The drawing under review shows one solid part. Ordinate dimensions are in mm from its lowest x, y, z. A direction names the side the tool comes from. Coordinates: 2 decimals unless noted, no trailing zeros. Loops run counter-clockwise (first coordinate to the right, second up) from the corner with the lowest first, then second, coordinate; pieces in that order, holes last. Notation, with made-up numbers: M -27,34.5 L 11,34.5 A34 cw 11,69.5 Z; hole C -7,11.25 d3. An arc over 180 degrees is marked long. Return JSON: item names as keys, results as strings.
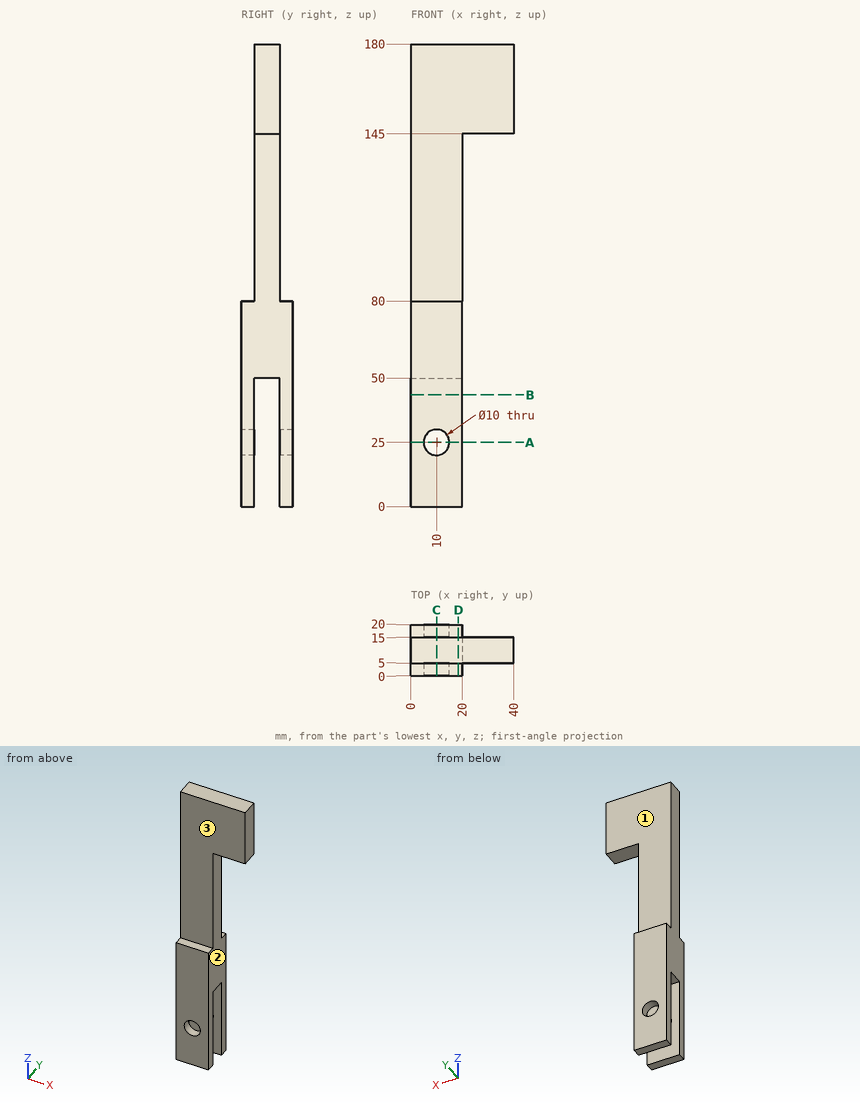
1. Add section A-A on z = 25. Give the boundary of the cut face in (x, y).
Check values:
{"outline": "M 0,0 L 5,0 L 5,5 L 0,5 Z; M 0,15 L 5,15 L 5,20 L 0,20 Z; M 15,0 L 20,0 L 20,5 L 15,5 Z; M 15,15 L 20,15 L 20,20 L 15,20 Z"}
2. Insertion check: pin 1 Ø2.5 at (x, y) = (10, 2.5) entering from +Z; pin 2 Ø11 at (x, y) = (30.5, 8) entering from -Z; pin 3 Ø3 at (y, z) = (5, 99) entering from +X. Each pin has a flat end and moves straight along its axis. Give the tip position at first contact, or say it passes through.
Check values:
{"pin 1": "z = 80", "pin 2": "z = 145", "pin 3": "x = 20"}
3. Add section C-C on x = 10. Give the boundary of the cut face in (y, z).
Check values:
{"outline": "M 0,0 L 5,0 L 5,20 L 0,20 Z; M 0,30 L 5,30 L 5,50 L 15,50 L 15,30 L 20,30 L 20,80 L 15,80 L 15,180 L 5,180 L 5,80 L 0,80 Z; M 15,0 L 20,0 L 20,20 L 15,20 Z"}
4. Machinability: for the marked faces 1, 2 and 3, which of the approach directions +Z, -Z, +X, -X, +Y, -Y give a long, thin tool a straight path to every point of the face, cutting with its end or side? Answer none if there is none.
Check values:
{"face 1": "+Z, +X, -X, +Y", "face 2": "-Z, +X, +Y, -Y", "face 3": "+Z, +X, -X, -Y"}
5. Add section B-B on z = 43.5. Give the boundary of the cut face in (x, y).
Check values:
{"outline": "M 0,0 L 20,0 L 20,5 L 0,5 Z; M 0,15 L 20,15 L 20,20 L 0,20 Z"}
6. To check wall thickness, follow line 1 (Z direction, x = 10, y = 17.95); line 2 (Y direction, x = 10, z = 111.5); line 3 (Z direction, x = 29.5, y = 12.5). State the ranges of each line that lie inside material, in increasing order.
Check values:
{"line 1": "0 to 20, 30 to 80", "line 2": "5 to 15", "line 3": "145 to 180"}
7. Add section D-D on x = 18.5. Give the boundary of the cut face in (y, z).
Check values:
{"outline": "M 0,0 L 5,0 L 5,50 L 15,50 L 15,0 L 20,0 L 20,80 L 15,80 L 15,180 L 5,180 L 5,80 L 0,80 Z"}
